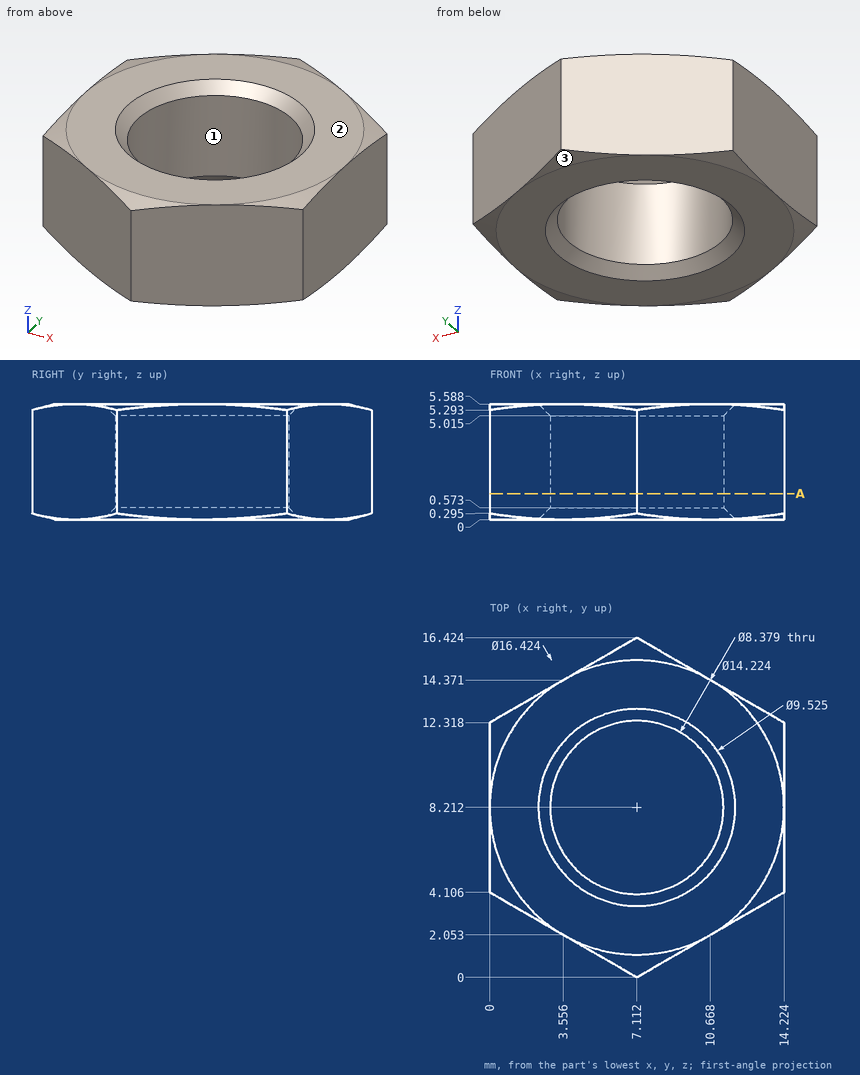
Check sheet for the drawn part. Datum: minimum x, y, z corner. Units: mm. Give positions to 0.01 mm unless a question says otherwise; leave off trailing zeros. Write each loop counter-clockwise with the first axis right and the second up, starting at its lowest first coordinate (ties: lowest second). Pieces come first, ordered by that corner, then holes.
(1) Mould release check, pull along Y, two halves, no side actions. Record for the marked faces 1, 2 and 3: +Y half, -Y half, draft (parallel to the pull), parting line (faces both ways), or undercut.
(2) Cross-section at A-A (z = 1.25). Enter the section's corners in (x, y) (1 decimal), plus the area to 3 significant figures.
(3) Material ranges on line 1 (X direction, y = 7.25, z = 1.8) (1 decimal); line 2 (Y direction, x = 10.25, z = 4.3) (1 decimal); line 3 (X direction, y = 10.75, z = 4.45) (1 decimal), recorded low to high.
(4) Gauge pin test, flat ends, axial feed: pin 1 (2 mm diameter, centred on x = 2.5, z = 3.5, fed in from +Y); pin 2 (1 mm diameter, centred on x = 12, z = 1, fed in from +Y). Record the tip position at first contact, or that the pin passes through.
Worked out:
1. face 1: undercut
1. face 2: draft
1. face 3: +Y half
2. outline: (0, 4.1) - (7.1, 0) - (14.2, 4.1) - (14.2, 12.3) - (7.1, 16.4) - (0, 12.3) - close; hole circle Ø8.4 at (7.1, 8.2)
2. area: 120 mm2
3. line 1: x = 0 to 3, 11.2 to 14.2
3. line 2: y = 1.8 to 5.4, 11 to 14.6
3. line 3: x = 0 to 3.8, 10.4 to 14.2
4. pin 1: stops at y = 14.34
4. pin 2: stops at y = 13.89
